For this review, use the dimensioned drawing (mm, ordinates from the lowest corner) and the shaded views. A direction names the side the tool comes from. Coordinates: 2 decimals unless noted, no trailing zeros. Loops run counter-clockwise (first coordinate to the right, second up) from the corner with the lowest first, then second, coordinate; pieces in that order, holes last.
1. Machinability: for the marked faces 4 and 5, which of the approach directions +Z, -Z, +X, -X, +Y, -Y give a long, thin tool a straight path to every point of the face, cutting with its end or side? Answer none if there is none.
2. Mouldability with a two-part tool opening along Z and no side actions: class the marked faces 1, 2 and 3 as pulls with the +Z half, pulls with the -Z half, needs draft (parallel to the pull), parting line crosses it, or undercut.
3. Take a section at A-A, the plane y = 26. State the section outline as (x, z) points.
4. To check wall thickness, follow probe 1 along Z at (x, y) = (2.95, 4.5); probe 2 along Z at (x, y) = (1.4, 32) (1 decimal); probe 3 along Z at (x, y) = (4.7, 5) (1 decimal). State the ranges of each line that lie inside material, in increasing order.
5. Clearance check with flat-ended pins moving along their axes: P1, Ø2, axis at x = 2.89, z = 2.5, coming from the +Y side; P2, Ø3, axis at y = 21.5, z = 1.5, coming from the +X side; P3, Ø1.5, axis at y = 12.5, z = 0.5, coming from the +X side; P4, Ø1, axis at x = 3.5, y = 10, coming from the -Z side. State where each tip first meets the part, or that it passes through.
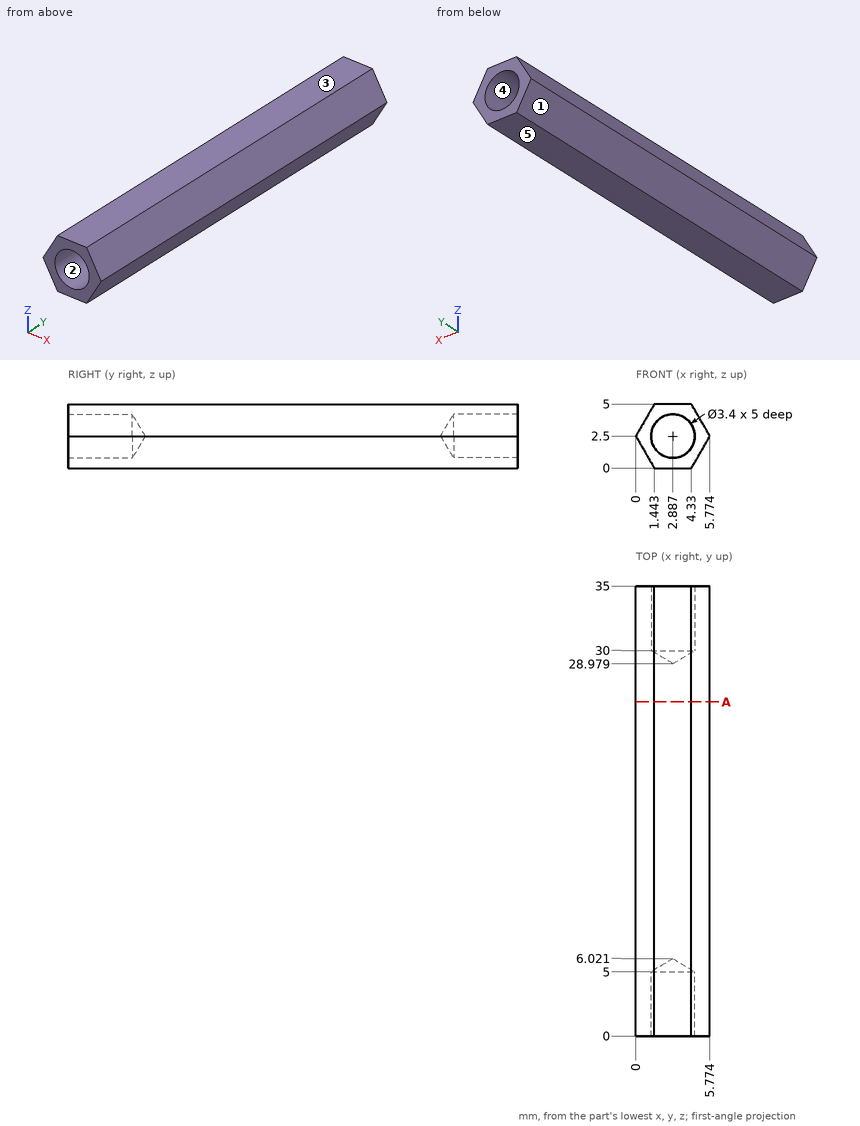
Results list:
1. face 4: +Y
1. face 5: -Z, +X, -X, +Y, -Y
2. face 1: pulls with the -Z half
2. face 2: undercut
2. face 3: pulls with the +Z half
3. outline: (0, 2.5) - (1.44, 0) - (4.33, 0) - (5.77, 2.5) - (4.33, 5) - (1.44, 5) - close
4. probe 1: z = 0 to 0.8, 4.2 to 5
4. probe 2: z = 0.1 to 1.7, 3.3 to 4.9
4. probe 3: z = 0.6 to 4.4
5. P1: stops at y = 29.58
5. P2: stops at x = 5.77
5. P3: stops at x = 5.05
5. P4: stops at z = 0
